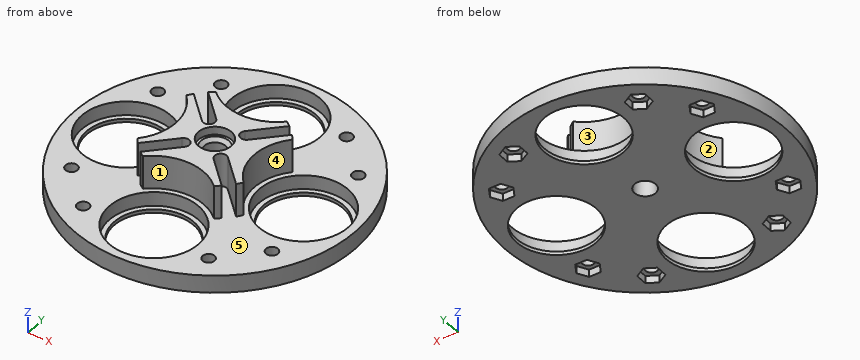
from build123d import *

# Parameters (mm, degrees)
SKETCH2_R           = 40
SKETCH2_R_2         = 11.33
SKETCH2_R_3         = 3
SKETCH2_R_4         = 1.7
BOSS_EXTRUDE1_DEPTH = 1
SKETCH3_R           = 40
SKETCH3_R_2         = 12.7
SKETCH3_R_3         = 3
SKETCH3_R_4         = 1.7
BOSS_EXTRUDE2_DEPTH = 4
SKETCH4_R           = 3
BOSS_EXTRUDE3_DEPTH = 9.5
SKETCH6_R           = 4.7
CUT_EXTRUDE2_DEPTH  = 2.3
CHAMFER1_SIZE       = 1
CUT_EXTRUDE1_DEPTH  = 2.1


with BuildPart() as part:
    # Sketch2 → Boss-Extrude1 (new body)
    with BuildSketch(Plane.XY):
        Circle(SKETCH2_R)
        with Locations((0, 25)):
            Circle(SKETCH2_R_2, mode=Mode.SUBTRACT)
        with Locations((25, 0)):
            Circle(SKETCH2_R_2, mode=Mode.SUBTRACT)
        with Locations((0, -25)):
            Circle(SKETCH2_R_2, mode=Mode.SUBTRACT)
        with Locations((-25, 0)):
            Circle(SKETCH2_R_2, mode=Mode.SUBTRACT)
        Circle(SKETCH2_R_3, mode=Mode.SUBTRACT)
        with Locations((17.697840613, 28.284271247)):
            Circle(SKETCH2_R_4, mode=Mode.SUBTRACT)
        with Locations((-17.697840613, 28.284271247)):
            Circle(SKETCH2_R_4, mode=Mode.SUBTRACT)
        with Locations((28.284271247, -17.697840613)):
            Circle(SKETCH2_R_4, mode=Mode.SUBTRACT)
        with Locations((28.284271247, 17.697840613)):
            Circle(SKETCH2_R_4, mode=Mode.SUBTRACT)
        with Locations((-17.697840613, -28.284271247)):
            Circle(SKETCH2_R_4, mode=Mode.SUBTRACT)
        with Locations((17.697840613, -28.284271247)):
            Circle(SKETCH2_R_4, mode=Mode.SUBTRACT)
        with Locations((-28.284271247, 17.697840613)):
            Circle(SKETCH2_R_4, mode=Mode.SUBTRACT)
        with Locations((-28.284271247, -17.697840613)):
            Circle(SKETCH2_R_4, mode=Mode.SUBTRACT)
    extrude(amount=BOSS_EXTRUDE1_DEPTH)

    # Sketch3 → Boss-Extrude2 (add)
    with BuildSketch(Plane.XY.offset(1)):
        Circle(SKETCH3_R)
        with Locations((0, 25)):
            Circle(SKETCH3_R_2, mode=Mode.SUBTRACT)
        with Locations((25, 0)):
            Circle(SKETCH3_R_2, mode=Mode.SUBTRACT)
        with Locations((0, -25)):
            Circle(SKETCH3_R_2, mode=Mode.SUBTRACT)
        with Locations((-25, 0)):
            Circle(SKETCH3_R_2, mode=Mode.SUBTRACT)
        Circle(SKETCH3_R_3, mode=Mode.SUBTRACT)
        with Locations((17.697840613, 28.284271247)):
            Circle(SKETCH3_R_4, mode=Mode.SUBTRACT)
        with Locations((-17.697840613, 28.284271247)):
            Circle(SKETCH3_R_4, mode=Mode.SUBTRACT)
        with Locations((28.284271247, -17.697840613)):
            Circle(SKETCH3_R_4, mode=Mode.SUBTRACT)
        with Locations((28.284271247, 17.697840613)):
            Circle(SKETCH3_R_4, mode=Mode.SUBTRACT)
        with Locations((-17.697840613, -28.284271247)):
            Circle(SKETCH3_R_4, mode=Mode.SUBTRACT)
        with Locations((17.697840613, -28.284271247)):
            Circle(SKETCH3_R_4, mode=Mode.SUBTRACT)
        with Locations((-28.284271247, 17.697840613)):
            Circle(SKETCH3_R_4, mode=Mode.SUBTRACT)
        with Locations((-28.284271247, -17.697840613)):
            Circle(SKETCH3_R_4, mode=Mode.SUBTRACT)
    extrude(amount=BOSS_EXTRUDE2_DEPTH)

    # Sketch4 → Boss-Extrude3 (add)
    with BuildSketch(Plane.XY.offset(5)):
        with BuildLine():
            Line((11.468948422, 13.873111478), (4.069996411, 6.474159467))
            ThreePointArc((4.069996411, 6.474159467), (4.069996411, 4.069996411), (6.474159467, 4.069996411))
            Line((6.474159467, 4.069996411), (13.873111478, 11.468948422))
            ThreePointArc((13.873111478, 11.468948422), (14.436174385, 10.751598445), (14.962183071, 10.006651675))
            ThreePointArc((14.962183071, 10.006651675), (10.955844123, 0), (14.962183071, -10.006651675))
            ThreePointArc((14.962183071, -10.006651675), (14.436174385, -10.751598445), (13.873111478, -11.468948422))
            Line((13.873111478, -11.468948422), (6.474159467, -4.069996411))
            ThreePointArc((6.474159467, -4.069996411), (4.069996411, -4.069996411), (4.069996411, -6.474159467))
            Line((4.069996411, -6.474159467), (11.468948422, -13.873111478))
            ThreePointArc((11.468948422, -13.873111478), (10.751598445, -14.436174385), (10.006651675, -14.962183071))
            ThreePointArc((10.006651675, -14.962183071), (0, -10.955844123), (-10.006651675, -14.962183071))
            ThreePointArc((-10.006651675, -14.962183071), (-10.751598445, -14.436174385), (-11.468948422, -13.873111478))
            Line((-11.468948422, -13.873111478), (-4.069996411, -6.474159467))
            ThreePointArc((-4.069996411, -6.474159467), (-4.069996411, -4.069996411), (-6.474159467, -4.069996411))
            Line((-6.474159467, -4.069996411), (-13.873111478, -11.468948422))
            ThreePointArc((-13.873111478, -11.468948422), (-14.436174385, -10.751598445), (-14.962183071, -10.006651675))
            ThreePointArc((-14.962183071, -10.006651675), (-10.955844123, 0), (-14.962183071, 10.006651675))
            ThreePointArc((-14.962183071, 10.006651675), (-14.436174385, 10.751598445), (-13.873111478, 11.468948422))
            Line((-13.873111478, 11.468948422), (-6.474159467, 4.069996411))
            ThreePointArc((-6.474159467, 4.069996411), (-4.069996411, 4.069996411), (-4.069996411, 6.474159467))
            Line((-4.069996411, 6.474159467), (-11.468948422, 13.873111478))
            ThreePointArc((-11.468948422, 13.873111478), (-10.751598445, 14.436174385), (-10.006651675, 14.962183071))
            ThreePointArc((-10.006651675, 14.962183071), (0, 10.955844123), (10.006651675, 14.962183071))
            ThreePointArc((10.006651675, 14.962183071), (10.751598445, 14.436174385), (11.468948422, 13.873111478))
        make_face()
        Circle(SKETCH4_R, mode=Mode.SUBTRACT)
    extrude(amount=BOSS_EXTRUDE3_DEPTH)

    # Sketch6 → Cut-Extrude2 (cut)
    with BuildSketch(Plane.XY.offset(14.5)):
        Circle(SKETCH6_R)
    extrude(amount=-CUT_EXTRUDE2_DEPTH, mode=Mode.SUBTRACT)

    # Chamfer1
    chamfer1_edges = [part.edges().sort_by_distance(p)[0] for p in [
        (-3, 0, 12.2),
    ]]
    chamfer(chamfer1_edges, length=CHAMFER1_SIZE)

    # Sketch5 → Cut-Extrude1 (cut)
    with BuildSketch(Plane(origin=(0, 0, 0), x_dir=(-1, 0, 0), z_dir=(0, 0, -1))):
        Polygon((29.929719515, 14.847840613), (31.575167782, 17.697840613), (29.929719515, 20.547840613), (26.63882298, 20.547840613), (24.993374713, 17.697840613), (26.63882298, 14.847840613), align=None)
        Polygon((-14.847840613, 29.929719515), (-17.697840613, 31.575167782), (-20.547840613, 29.929719515), (-20.547840613, 26.63882298), (-17.697840613, 24.993374713), (-14.847840613, 26.63882298), align=None)
        Polygon((20.547840613, 26.63882298), (20.547840613, 29.929719515), (17.697840613, 31.575167782), (14.847840613, 29.929719515), (14.847840613, 26.63882298), (17.697840613, 24.993374713), align=None)
        Polygon((26.63882298, -20.547840613), (29.929719515, -20.547840613), (31.575167782, -17.697840613), (29.929719515, -14.847840613), (26.63882298, -14.847840613), (24.993374713, -17.697840613), align=None)
        Polygon((14.847840613, -29.929719515), (17.697840613, -31.575167782), (20.547840613, -29.929719515), (20.547840613, -26.63882298), (17.697840613, -24.993374713), (14.847840613, -26.63882298), align=None)
        Polygon((-20.547840613, -26.63882298), (-20.547840613, -29.929719515), (-17.697840613, -31.575167782), (-14.847840613, -29.929719515), (-14.847840613, -26.63882298), (-17.697840613, -24.993374713), align=None)
        Polygon((-29.929719515, -14.847840613), (-31.575167782, -17.697840613), (-29.929719515, -20.547840613), (-26.63882298, -20.547840613), (-24.993374713, -17.697840613), (-26.63882298, -14.847840613), align=None)
        Polygon((-26.63882298, 20.547840613), (-29.929719515, 20.547840613), (-31.575167782, 17.697840613), (-29.929719515, 14.847840613), (-26.63882298, 14.847840613), (-24.993374713, 17.697840613), align=None)
    extrude(amount=-CUT_EXTRUDE1_DEPTH, mode=Mode.SUBTRACT)


solid = part.part
For this review, take the finished solid that the model builds, in its own axes (mm). Face numbers are marked on the shaded views. A direction names the side the tool comes from. Give positions to 0.01 mm unless a question says otherwise; leave off trailing zeros. Loops run counter-clockwise (first coordinate to the right, second up) from the corner with the lowest first, then second, coordinate; pieces in that order, holes last.
Item 1: Insertion check: pin 1 (2 mm diameter, centred on x = 19.5, z = 2.5, fed in from +Y); pin 2 (2.5 mm diameter, centred on x = 28.28, y = -17.7, fed in from +Z); pin 3 (23 mm diameter, centred on x = 0, y = 25, fed in from -Z); pin 4 (2.5 mm diameter, centred on y = -28, z = 1.5, fed in from +X). Each pin has a flat end and moves straight along its axis. Give the tip position at first contact, or say it passes through.
Item 2: Tool access review of the marked faces 1, 2, 3, 4 and 5: name each direction out of +Z, -Z, +X, -X, +Y, -Y from which nothing blocks a thin tool from reaching the whole face with its end or side.
Item 3: Take a section at D-D, the plane y = 34. State the section outline as (x, z) points.
Item 4: For line 1 along Y through (x, z) = (0, 0.75); line 2 along Y through (x, z) = (0, 2.8); line 3 along X through (y, z) = (7, 10), list the stretches that pass through material, from the lowest coordinate up.
Item 5: Take a section at C-C, the plane x = 35. State the section outline as (y, z) points.
Item 6: Take a section at A-A, the plane x = 0. Give the number of separate pieces and of enclosed holes in the cut face, and give its area (3 significant figures).
Calculated:
1. pin 1: stops at y = 35.46
1. pin 2: passes through
1. pin 3: stops at z = 0
1. pin 4: stops at x = 29.74
2. face 1: +Z, -Y
2. face 2: +Z, -X
2. face 3: +Z, +Y
2. face 4: +Z, +X
2. face 5: +Z
3. outline: (-21.07, 0) - (-6.88, 0) - (-6.88, 1) - (-8.96, 1) - (-8.96, 5) - (-21.07, 5) - close; (6.88, 0) - (21.07, 0) - (21.07, 5) - (8.96, 5) - (8.96, 1) - (6.88, 1) - close
4. line 1: y = -40 to -36.33, -13.67 to -3, 3 to 13.67, 36.33 to 40
4. line 2: y = -40 to -37.7, -12.3 to -3, 3 to 12.3, 37.7 to 40
4. line 3: x = -12.76 to -9.4, -4.6 to 4.6, 9.4 to 12.76
5. outline: (-19.36, 0) - (-5.33, 0) - (-5.33, 1) - (-7.83, 1) - (-7.83, 5) - (-19.36, 5) - close; (5.33, 0) - (19.36, 0) - (19.36, 5) - (7.83, 5) - (7.83, 1) - (5.33, 1) - close
6. separate pieces: 4
6. enclosed holes: 0
6. area: 264 mm2
